Check sheet for the modelled part. Datum: model origin and axes. Units: mm. Round coordinates to 2 decimals unless told otherwise and drop trailing zeros. Loops run counter-clockwise (first coordinate to the right, second up) from the corner with the lowest first, then second, coordinate; pieces in that order, holes last. Notation, with made-up numbers: (83, 35) - (103, 35) arc R8 cw to (103, 43) - close; hole circle Ø7 at (59.5, 81.5). An arc over 180 degrees is marked (long way). Return JSON: item names as keys, results as strings.
from build123d import *

# Parameters (mm, degrees)
BOSS_EXTRUDE1_DEPTH = 3
FILLET2_R           = 0.1


with BuildPart() as part:
    # Sketch1 → Boss-Extrude1 (new body)
    with BuildSketch(Plane.XY):
        Polygon((-1.25, -12.5), (1.25, -9.5), (1.25, 7.5), (-1.25, 7.5), align=None)
    extrude(amount=BOSS_EXTRUDE1_DEPTH)

    # Fillet2
    fillet2_edges = [part.edges().sort_by_distance(p)[0] for p in [
        (-1.25, -12.5, 1.5),
    ]]
    fillet(fillet2_edges, radius=FILLET2_R)


solid = part.part
Q1. Sectioned sample at A-A (z = 1.95). Enter the section's corners in (x, y), plus the area to 3 significant figures.
Answer key:
{"outline": "(-1.25, -12.22) arc R0.1 ccw to (-1.07, -12.29) - (1.25, -9.5) - (1.25, 7.5) - (-1.25, 7.5) - close", "area": "46.2 mm²"}
Q2. Sectioned sample at B-B (x = 1). Enter the section's corners in (y, z).
Answer key:
{"outline": "(-9.8, 0) - (7.5, 0) - (7.5, 3) - (-9.8, 3) - close"}
Q3. Scan lines: probe 1 along Y at (x, z) = (-0.95, 2.15); probe 2 along Y at (x, z) = (0.7, 1.1); probe 3 along X at (y, z) = (-11.25, 2.5). Record each from-to range of solid material in increasing order. Write a range as [from, to].
Answer key:
{"probe 1": "y = [-12.14, 7.5]", "probe 2": "y = [-10.16, 7.5]", "probe 3": "x = [-1.25, -0.21]"}
Q4. Sectioned sample at C-C (y = -10). Enter the section's corners in (x, z).
Answer key:
{"outline": "(-1.25, 0) - (0.83, 0) - (0.83, 3) - (-1.25, 3) - close"}
